Could you check a few things on this drawing? It's one solid part, dimensions in mm from its lowest x, y, z. Round coordinates to 2 decimals unless told otherwise and drop trailing zeros. Write each loop counter-clockwise with the first axis right and the second up, starting at its lowest first coordinate (ties: lowest second). Pieces come first, ordered by that corner, then holes. Notation, with made-up numbers: (12.25, 14) - (52.25, 14) arc R26 ccw to (52.25, 40) - close; hole circle Ø5 at (60.25, -29.5). An arc over 180 degrees is marked (long way). Use one line per item in the form item = value. Start each with the question number.
1. Will these pins go through, and if not, where does the flat tip stop? pin 1 (8 mm diameter, centred on y = 202.5, z = 10, fed in from -X); pin 2 (12.5 mm diameter, centred on x = 97.5, y = 525.5, fed in from -Z); pin 3 (5 mm diameter, centred on x = 166.5, z = 3.5, fed in from -Y); pin 4 (5 mm diameter, centred on x = 120, z = 2.5, fed in from -Y).
2. I want a section at A-A, the plane x = 45.5. List the corners of the cut face in (y, z) for me.
3. If I drill on line 1 along Y through (x, z) = (69, 2.75); line 2 along Y through (x, z) = (160, 12); line 3 along Y through (x, z) = (172.5, 5), over which ranges is the centre line in solid material (lowest first)?
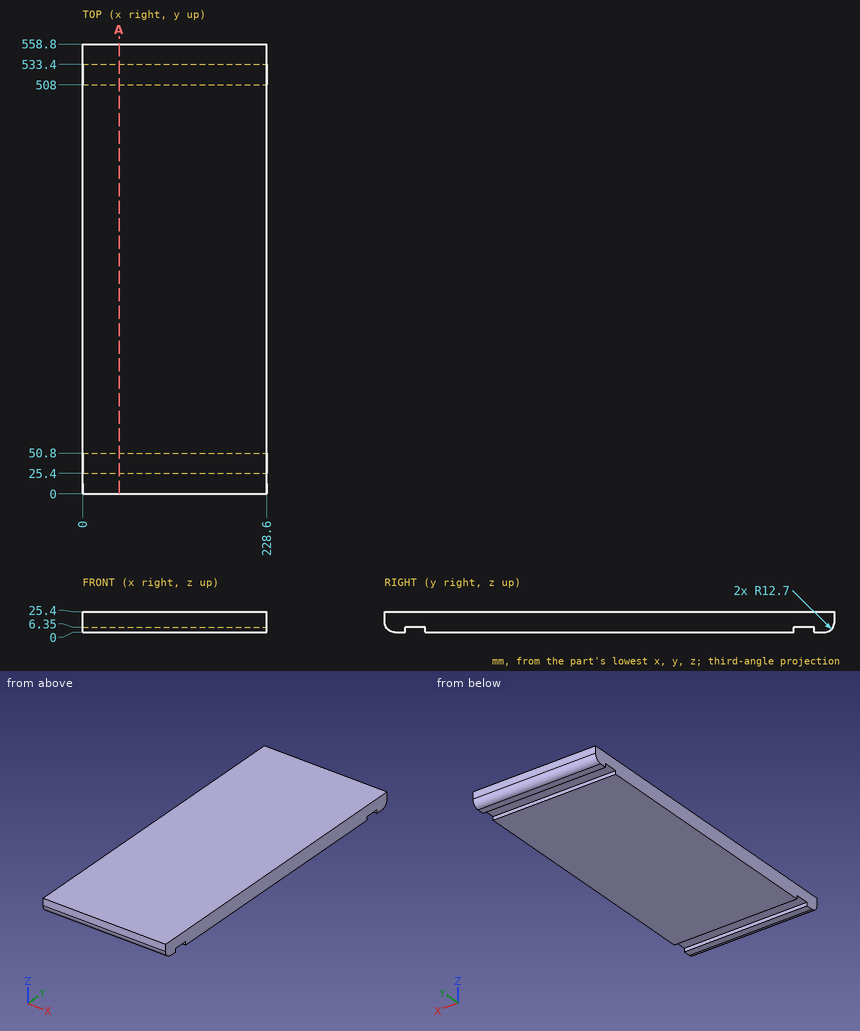
Model answer:
q1.pin_1 = 0
q1.pin_2 = 6.35
q1.pin_3 = 1.91
q1.pin_4 = 2.6
q2.outline = (0, 12.7) arc R12.7 ccw to (12.7, 0) - (25.4, 0) - (25.4, 6.35) - (50.8, 6.35) - (50.8, 0) - (508, 0) - (508, 6.35) - (533.4, 6.35) - (533.4, 0) - (546.1, 0) arc R12.7 ccw to (558.8, 12.7) - (558.8, 25.4) - (0, 25.4) - close
q3.line_1 = 4.81 to 25.4, 50.8 to 508, 533.4 to 553.99
q3.line_2 = 0.02 to 558.78
q3.line_3 = 2.6 to 25.4, 50.8 to 508, 533.4 to 556.2
